Read the model definition and answer for the solid it produces. Units are mm, in the model's axes. A direction names the side the tool comes from. Coordinates: 2 decimals unless noted, no trailing zeros. Order: outer loops, then holes, each group sorted by start corner. A loop starts at its lowest first (then second) coordinate and runs counter-clockwise, first axis right, second up. Notation, with made-up numbers: (33.5, -13) -> (66.5, -13) arc R12 cw to (66.5, 10) -> close; hole circle Ø7 at (-29.5, 9.25). An arc over 180 degrees is marked (long way). Answer as a JSON object with one key per item and string values. Group by question number.
1) Consider L1, parallel to Z at x = 1.9, y = 0; L2, parallel to Z at x = 2.65, y = -3; L3, parallel to Y at x = 2.15, z = -0.5. Determine where each line is inside the solid, lowest interval first.
2) A tool of negligible diameter and unlimited length cuts with its end or side. For faces 4 (the flat face through (2, 8, -4)), 5 (the flat face through (2, -8, 0)), from which of +Z, -Z, +X, -X, +Y, -Y can it reach the whole face along a straight path? Write none if from no direction.
3) Section D-D on z = -6.75 is taken. Determine the outline of the cut face in (x, y), and give its area (3 significant figures).
4) Section A-A on y = 0 is taken. Determine the outline of the cut face in (x, z).
5) Section B-B on x = 2.3 is taken. Determine the outline of the cut face in (y, z), and give its area (3 significant figures).
6) Given pin 1 (1.6 mm diameter, centred on x = 1, y = 9.5, fed in from -Z); pin 2 (9 mm diameter, centred on y = 0, z = 0, fed in from -X) (3 decimals), each flat-ended and moving along its own axis, determine where each tip first touches the part or whether it passes through.
7) Determine the mould class of faces 1 (the flat face through (2, 10, 0)), 2 (the flat face through (3.25, 4, 4)), 3 (the cylindrical face through (1.6, -1.08, 4.88)) for opening direction Z: released by +Z, released by -Z, zero draft, split by the parting line, or undercut.
8) Section C-C on z = -0.5 is taken. Determine the outline of the cut face in (x, y), and give its area (3 significant figures).
Autodesk Inventor part; units mm, degrees
ref_plane "YZ Plane" through (0, 0, 0) normal (1, 0, 0) x (0, 1, 0)
ref_plane "XZ Plane" through (0, 0, 0) normal (0, 1, 0) x (-1, 0, 0)
ref_plane "XY Plane" through (0, 0, 0) normal (0, 0, 1) x (1, 0, 0)
sketch "Sketch1" plane through (0, 0, 0) normal (1, 0, 0) x (0, 1, 0)
  line L0 (-92.7646, -8.503) -> (-89.7646, -8.503)
  line L1 (-89.7646, -8.503) -> (-89.7646, -11.753)
  line L2 (-89.7646, -11.753) -> (-92.7646, -11.753)
  line L3 (-92.7646, -11.753) -> (-92.7646, -8.503)
  line L4 (-92.7646, -21.6527) -> (-89.7646, -21.6527)
  line L5 (-89.7646, -21.6527) -> (-89.7646, -21.7527)
  line L6 (-89.7646, -21.7527) -> (-92.7646, -21.7527)
  line L7 (-92.7646, -21.7527) -> (-92.7646, -21.6527)
  circle A0 centre (0, 0) radius 5
  line L8 (-8, -8) -> (8, -8)
  line L9 (8, -8) -> (8, 8)
  line L10 (8, 8) -> (-8, 8)
  line L11 (-8, 8) -> (-8, -8)
  line L12 (-8, 0) -> (8, 0) construction
  line L13 (0, 8) -> (0, -8) construction
  line L14 (8, 8) -> (11.25, 8)
  line L15 (11.25, 8) -> (11.25, 0)
  line L16 (11.25, 0) -> (8, 0)
  line L17 (8, 0) -> (8, 8)
  dimension "d0" = 3
  dimension "mat" = 3.25
  dimension "d2" = 3
  dimension "kerf" = 0.1
  dimension "d22" = 10
  dimension "d23" = 16
  dimension "d24" = 16
  dimension "d25" = 3.25
  dimension "d26" = 8
extrude "Extrusion3" add sketch "Sketch1" along normal blind 3.25 contours L11 L10 L9 L8 | L9 L14 L15 L16
equation "\"d25\" = mat"
equation "\"d27\" = mat"
properties part number "body-side2"
Worked answers:
{
 "1": {"L1": "z = -8 to -5, 5 to 8", "L2": "z = -8 to -4, 4 to 8", "L3": "y = -8 to -4.97, 4.97 to 8"},
 "2": {"face 4": "-Z, +X, -X, +Y", "face 5": "+Z, -Z, +X, -X, -Y"},
 "3": {"outline": "(0, -8) -> (3.25, -8) -> (3.25, 8) -> (0, 8) -> close", "area": "52.0 mm²"},
 "4": {"outline": "(0, -8) -> (3.25, -8) -> (3.25, -5) -> (0, -5) -> close; (0, 5) -> (3.25, 5) -> (3.25, 8) -> (0, 8) -> close"},
 "5": {"outline": "(-8, -8) -> (8, -8) -> (8, 0) -> (11.25, 0) -> (11.25, 8) -> (-8, 8) -> close; hole circle Ø10 at (0, 0)", "area": "203 mm²"},
 "6": {"pin 1": "stops at z = 0", "pin 2": "passes through"},
 "7": {"face 1": "released by -Z", "face 2": "zero draft", "face 3": "undercut"},
 "8": {"outline": "(0, -8) -> (3.25, -8) -> (3.25, -4.97) -> (0, -4.97) -> close; (0, 4.97) -> (3.25, 4.97) -> (3.25, 8) -> (0, 8) -> close", "area": "19.7 mm²"}
}
